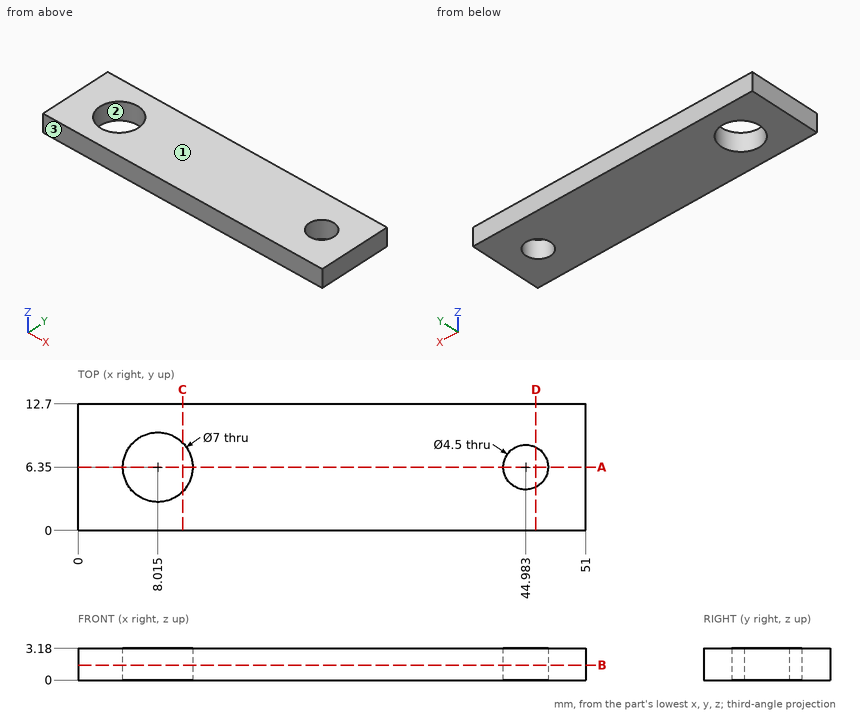
Source: three-view drawing plus pictorial views. Frame: mm from the lowest corner of the part. Coordinates: 2 decimals unless noted, no trailing zeros. Order: outer loops, then holes, each group sorted by start corner. A loop starts at its lowest first (then second) coordinate and runs counter-clockwise, first axis right, second up.
1) Draft query along Y for the marked faces 1, 2 and 3. Return one class per face: released by +Y, released by -Y, zero draft, split by the parting line, or undercut.
Result sheet:
face 1: zero draft
face 2: undercut
face 3: released by -Y
2) Section A-A (y = 6.35). Return loops of the section in (x, z) (1 decimal), then the cut area to 3 significant figures.
Result sheet:
outline: (0, 0) - (4.5, 0) - (4.5, 3.2) - (0, 3.2) - close; (11.5, 0) - (42.7, 0) - (42.7, 3.2) - (11.5, 3.2) - close; (47.2, 0) - (51, 0) - (51, 3.2) - (47.2, 3.2) - close
area: 126 mm2
3) Section D-D (x = 46). Return loops of the section in (y, z).
Result sheet:
outline: (0, 0) - (4.34, 0) - (4.34, 3.18) - (0, 3.18) - close; (8.36, 0) - (12.7, 0) - (12.7, 3.18) - (8.36, 3.18) - close
4) Section C-C (x = 10.5). Return loops of the section in (y, z) (1 decimal), then the cut area to 3 significant figures.
Result sheet:
outline: (0, 0) - (3.9, 0) - (3.9, 3.2) - (0, 3.2) - close; (8.8, 0) - (12.7, 0) - (12.7, 3.2) - (8.8, 3.2) - close
area: 24.7 mm2
5) Ray query, probe 1 along X at (y, z) = (6.25, 2.6) (1 decimal); probe 2 along X at (y, z) = (5, 3) (1 decimal); probe 3 along X at (y, z) = (9.5, 2.2) (1 decimal). Return the intervals inside material, ascending.
Result sheet:
probe 1: x = 0 to 4.5, 11.5 to 42.7, 47.2 to 51
probe 2: x = 0 to 4.8, 11.2 to 43.2, 46.8 to 51
probe 3: x = 0 to 6.5, 9.5 to 51
6) Section B-B (z = 1.5). Give the number of separate pieces and of enclosed holes in the cut face, then the cut area to 3 significant figures.
Result sheet:
separate pieces: 1
enclosed holes: 2
area: 593 mm2
